```python
from build123d import *

# Parameters (mm, degrees)
F0_W     = 50
F0_H     = 90
F1_DEPTH = 100
F2_T     = -0.4
F4_DEPTH = 59


with BuildPart() as f1:
    # F0 (on Front) → F1 (new body)
    with BuildSketch(Plane.XZ):
        with Locations((25, 45)):
            Rectangle(F0_W, F0_H)
    extrude(amount=-F1_DEPTH)

    # F2
    f2_openings = [f1.faces().sort_by_distance(p)[0] for p in [
        (25, 100, 45),
    ]]
    offset(amount=F2_T, openings=f2_openings)

    # F3 (on face) → F4 (cut)
    with BuildSketch(Plane.XY.offset(90)):
        Polygon((24, 29), (50, 0), (50, 71), (24, 71), align=None)
    extrude(amount=-F4_DEPTH, mode=Mode.SUBTRACT)


solid = f1.part
```
Here's how the part is built. I have some questions about the finished solid (model axes, mm). A direction names the side the tool comes from. Give positions to 0.01 mm unless a question says otherwise; leave off trailing zeros. Loops run counter-clockwise (first coordinate to the right, second up) from the corner with the lowest first, then second, coordinate; pieces in that order, holes last. Notation, with made-up numbers: (44.5, 18) -> (71.5, 18) arc R27 cw to (71.5, 35) -> close; hole circle Ø7 at (-2.5, 13). An arc over 180 degrees is marked (long way). Use one line per item in the form item = value. Start each with the question number.
1) Please list where these lines run through material, in increasing order: line 1 along Z through (x, y) = (44, 78); line 2 along X through (y, z) = (88, 71.5); line 3 along X through (y, z) = (17, 38.5).
2) For P1, Ø10, axis at y = 49, z = 60, coming from the +X side; P2, Ø1, axis at x = 41, z = 73.5, coming from the +Y side, each with a flat end and sliding along its axis, tell me the tip position at first contact or that it passes through.
3) Imagine slicing it at C-C (x = 10). Please give me the cut outline in (y, z).
4) Imagine slicing it at D-D (z = 19). Please give me the cut outline in (x, y).
5) Imagine slicing it at B-B (z = 45). Please give me the cut outline in (x, y), then the cut area to 3 significant figures.
6) Thinking about a two-plate mould opening in Z: for faces 3 (the face through (19, 49, 90)), 4 (the face through (25, 0.4, 46)), 5 (the face through (25, 49, 0)), 6 (the face through (50, 60, 24)), which applies, +Z half, -Z half, draft (parallel to the pull), parting line (faces both ways), or undercut?
7) Which directions (+Z, -Z, +X, -X, +Y, -Y) give clear straight access to the entire face, cutting with the end or side of a thin tool? Please do faces 1 (the face through (0, 49, 44)), 2 (the face through (49.6, 61, 25)).
8) Imagine slicing it at A-A (y = 85). Please give me the cut outline in (x, z), then the cut area to 3 significant figures.
Check values:
q1.line_1 = 0 to 0.4, 89.6 to 90
q1.line_2 = 0 to 0.4, 49.6 to 50
q1.line_3 = 0 to 0.4
q2.P1 = 0.4
q2.P2 = 0.4
q3.outline = (0, 0) -> (100, 0) -> (100, 0.4) -> (0.4, 0.4) -> (0.4, 89.6) -> (100, 89.6) -> (100, 90) -> (0, 90) -> close
q4.outline = (0, 0) -> (50, 0) -> (50, 100) -> (49.6, 100) -> (49.6, 0.4) -> (0.4, 0.4) -> (0.4, 100) -> (0, 100) -> close
q5.outline = (0, 0) -> (50, 0) -> (49.6, 0.45) -> (49.6, 0.4) -> (0.4, 0.4) -> (0.4, 100) -> (0, 100) -> close; (49.6, 71) -> (50, 71) -> (50, 100) -> (49.6, 100) -> close
q5.area = 71.4 mm^2
q6.face_3 = +Z half
q6.face_4 = undercut
q6.face_5 = -Z half
q6.face_6 = draft
q7.face_1 = +Z, -Z, -X, +Y, -Y
q7.face_2 = +Y
q8.outline = (0, 0) -> (50, 0) -> (50, 90) -> (0, 90) -> close; hole (0.4, 0.4) -> (49.6, 0.4) -> (49.6, 89.6) -> (0.4, 89.6) -> close
q8.area = 111 mm^2
